Could you check a few things on this drawing? It's one solid part, dimensions in mm from its lowest x, y, z. A direction names the side the tool comes from. Give positions to 0.01 mm unless a question says otherwise; leave off trailing zeros. Order: outer loops, then holes, each group sorted by start corner. A loop starts at its lowest first (then second) coordinate and runs counter-clockwise, first axis right, second up. Notation, with made-up numbers: (79.5, 50) - (90.5, 50) arc R22 cw to (90.5, 69) - close; hole circle Ø7 at (79.5, 67.25). An arc over 180 degrees is marked (long way). Answer as CSV lines item,"result".
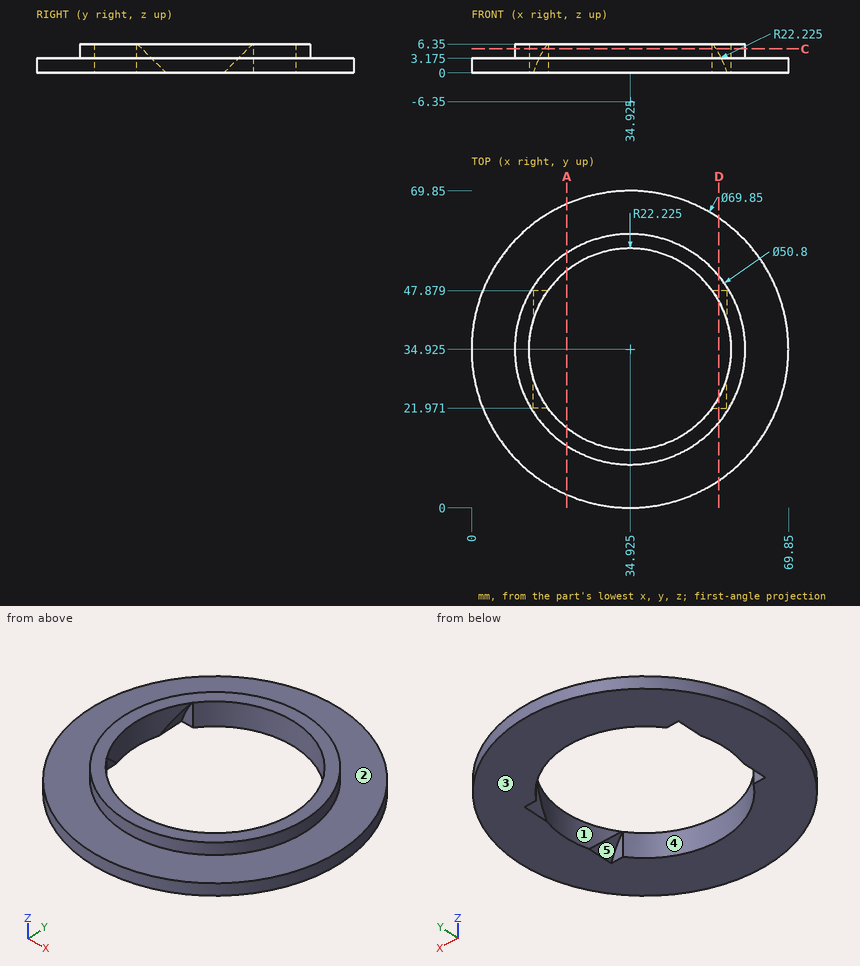
1) Which directions (+Z, -Z, +X, -X, +Y, -Y) give clear straight access to the entire face, cutting with the end or side of a thin tool? Please do the marked faces 3, 4 and 5.
Answer block:
face 3,"-Z, +X, -X, +Y, -Y"
face 4,"+Z, -Z"
face 5,"-Z"
2) I want a section at C-C on z = 5.25. Write out the boundary of the cut face in (x, y) (3 decimals), plus the area to 3 significant figures.
Answer block:
outline,"circle Ø50.8 at (34.925, 34.925); hole (15.967, 21.971) - (16.866, 21.971) arc R22.225 ccw to (52.984, 21.971) - (53.883, 21.971) - (53.883, 23.325) arc R22.225 ccw to (53.883, 46.525) - (53.883, 47.879) - (52.984, 47.879) arc R22.225 ccw to (16.866, 47.879) - (15.967, 47.879) - (15.967, 46.525) arc R22.225 ccw to (15.967, 23.325) - close"
area,"473 mm2"
3) I'm going to push flat-ended pins straight in: P1, Ø1, axis at x = 44, z = 3.5, coming from the -Y side; P2, Ø6, axis at x = 32, y = 14, coming from the +Z side; P3, Ø3, axis at y = 26.5, z = 5, coming from the +X side; P4, Ø1.6, axis at x = 55, z = 3, coming from the -Y side. Where does each tip first touch, or does it pass through?
Answer block:
P1,"y = 1.1"
P2,"z = 6.35"
P3,"x = 59.36"
P4,"y = 5.8"
4) I need wall thicknesses on line 1 along Z through (x, y) = (59.5, 45.5) (3 decimals); line 2 along X through (y, z) = (33, 0.5); line 3 along Y through (x, z) = (50, 4.25). Which ranges of each line are inside material? Lowest first, please. Write a range as [from, to].
Answer block:
line 1,"[0, 3.175]"
line 2,"[0.05, 12.78], [57.07, 69.8]"
line 3,"[14.48, 18.59], [51.26, 55.37]"
5) I want a section at A-A on x = 21. Write out the boundary of the cut face in (y, z) (3 decimals), plus the area to 3 significant figures.
Answer block:
outline,"(2.896, 0) - (17.603, 0) - (17.603, 6.35) - (13.682, 6.35) - (13.682, 3.175) - (2.896, 3.175) - close; (52.247, 0) - (66.954, 0) - (66.954, 3.175) - (56.168, 3.175) - (56.168, 6.35) - (52.247, 6.35) - close"
area,"118 mm2"
6) I want a section at D-D on x = 54.5. Write out the boundary of the cut face in (y, z) (3 decimals), plus the area to 3 significant figures.
Answer block:
outline,"(6.001, 0) - (21.971, 0) - (21.971, 4.175) - (24.4, 4.175) - (24.4, 6.35) - (18.739, 6.35) - (18.739, 3.175) - (6.001, 3.175) - close; (45.45, 4.175) - (47.879, 4.175) - (47.879, 0) - (63.849, 0) - (63.849, 3.175) - (51.111, 3.175) - (51.111, 6.35) - (45.45, 6.35) - close"
area,"132 mm2"
7) If we mould it in two halves opening along Y, with no side actions, what happens to the marked faces 1 and 2? For each: +Y half, -Y half, draft (parallel to the pull), parting line (faces both ways), or undercut.
Answer block:
face 1,"undercut"
face 2,"draft"
